from build123d import *

# Parameters (mm, degrees)
F0_W     = 100
F0_H     = 40
F1_DEPTH = 3
F2_R     = 3.685803
F3_DEPTH = 25


with BuildPart() as f1:
    # F0 (on Top) → F1 (new body)
    with BuildSketch(Plane.XY):
        Rectangle(F0_W, F0_H)
    extrude(amount=F1_DEPTH)

    # F2 (on face) → F3 (cut)
    with BuildSketch(Plane.XY.offset(3)):
        with Locations((-43.042492, -13.054423)):
            Circle(F2_R)
        with Locations((-43.099029, -4.054601)):
            Circle(F2_R)
        with Locations((-43.155565, 4.945222)):
            Circle(F2_R)
        with Locations((-43.212102, 13.945044)):
            Circle(F2_R)
        with Locations((-33.155565, 4.945222)):
            Circle(F2_R)
        with Locations((-33.212102, 13.945044)):
            Circle(F2_R)
        with Locations((-33.099029, -4.054601)):
            Circle(F2_R)
        with Locations((-33.042492, -13.054423)):
            Circle(F2_R)
        with Locations((-23.042492, -13.054423)):
            Circle(F2_R)
        with Locations((-23.099029, -4.054601)):
            Circle(F2_R)
        with Locations((-23.212102, 13.945044)):
            Circle(F2_R)
        with Locations((-23.155565, 4.945222)):
            Circle(F2_R)
        with Locations((-13.099029, -4.054601)):
            Circle(F2_R)
        with Locations((-13.042492, -13.054423)):
            Circle(F2_R)
        with Locations((-3.042492, -13.054423)):
            Circle(F2_R)
        with Locations((-3.099029, -4.054601)):
            Circle(F2_R)
        with Locations((-13.155565, 4.945222)):
            Circle(F2_R)
        with Locations((-13.212102, 13.945044)):
            Circle(F2_R)
        with Locations((-3.212102, 13.945044)):
            Circle(F2_R)
        with Locations((-3.155565, 4.945222)):
            Circle(F2_R)
        with Locations((6.957508, -13.054423)):
            Circle(F2_R)
        with Locations((6.900971, -4.054601)):
            Circle(F2_R)
        with Locations((6.844435, 4.945222)):
            Circle(F2_R)
        with Locations((6.787898, 13.945044)):
            Circle(F2_R)
        with Locations((16.957508, -13.054423)):
            Circle(F2_R)
        with Locations((16.900971, -4.054601)):
            Circle(F2_R)
        with Locations((16.844435, 4.945222)):
            Circle(F2_R)
        with Locations((16.787898, 13.945044)):
            Circle(F2_R)
        with Locations((26.957508, -13.054423)):
            Circle(F2_R)
        with Locations((26.900971, -4.054601)):
            Circle(F2_R)
        with Locations((26.844435, 4.945222)):
            Circle(F2_R)
        with Locations((36.900971, -4.054601)):
            Circle(F2_R)
        with Locations((36.957508, -13.054423)):
            Circle(F2_R)
        with Locations((36.844435, 4.945222)):
            Circle(F2_R)
        with Locations((36.787898, 13.945044)):
            Circle(F2_R)
        with Locations((26.787898, 13.945044)):
            Circle(F2_R)
    extrude(amount=-F3_DEPTH, mode=Mode.SUBTRACT)


solid = f1.part
Read the model definition and answer for the solid it produces. Units are mm, in the model's axes. Round coordinates to 2 decimals unless told otherwise and drop trailing zeros. Write each loop counter-clockwise with the first axis right and the second up, starting at its lowest first coordinate (ties: lowest second). Pieces come first, ordered by that corner, then holes. Notation, with made-up numbers: M -31.5,81 L 19.5,81 A25 ccw 19.5,103 Z; hole C -3.5,74 d6. An arc over 180 degrees is marked long. Use a Markdown table: item, result.
1) For a pull along Y with two mould halves and no side action, classify faces 1 (the flat face through (10, 0, 0)), 2 (the cylindrical face through (-3.842, -16.653, 1.521)) as pulls with the +Y half, pulls with the -Y half, needs draft (parallel to the pull), parting line crosses it, or undercut.
Answers follow:
| item | result |
|---|---|
| face 1 | needs draft |
| face 2 | undercut |
2) The part is cut by section B-B (x = -2). Write down the section's boundary in (y, z), plus the area to 3 significant figures.
Answers follow:
| item | result |
|---|---|
| outline | M -20,0 L -16.59,0 L -16.59,3 L -20,3 Z; M -9.52,0 L -7.57,0 L -7.57,3 L -9.52,3 Z; M -0.54,0 L 1.45,0 L 1.45,3 L -0.54,3 Z; M 8.45,0 L 10.46,0 L 10.46,3 L 8.45,3 Z; M 17.43,0 L 20,0 L 20,3 L 17.43,3 Z |
| area | 35.8 mm2 |
3) The part is cut by section A-A (x = 37.5). Write down the section's boundary in (y, z), plus the area to 3 significant figures.
Answers follow:
| item | result |
|---|---|
| outline | M -20,0 L -16.7,0 L -16.7,3 L -20,3 Z; M -9.41,0 L -7.69,0 L -7.69,3 L -9.41,3 Z; M -0.42,0 L 1.32,0 L 1.32,3 L -0.42,3 Z; M 8.57,0 L 10.33,0 L 10.33,3 L 8.57,3 Z; M 17.56,0 L 20,0 L 20,3 L 17.56,3 Z |
| area | 32.8 mm2 |
4) The part is cut by section C-C (z = 2.4). Give the number of separate pieces and of enclosed holes in the cut face, plus the area to 3 significant figures.
Answers follow:
| item | result |
|---|---|
| separate pieces | 1 |
| enclosed holes | 36 |
| area | 2,460 mm2 |
5) Straight lines are drawn through the part: line 1 along Y through (x, z) = (7, 2.4); line 2 along Y through (x, z) = (-45, 1.15). For each, find the intervals that lie inside material, in ascending order. Write a range as [from, to].
Answers follow:
| item | result |
|---|---|
| line 1 | y = [-20, -16.74], [-9.37, -7.74], [-0.37, 1.26], [8.63, 10.27], [17.62, 20] |
| line 2 | y = [-20, -16.18], [-9.93, -7.21], [-0.9, 1.75], [8.14, 10.72], [17.17, 20] |
